Check sheet for the modelled part. Datum: model origin and axes. Units: mm. Face numbers are marked on the shaded views. Coordinates: 2 decimals unless noted, no trailing zeros. Write each loop counter-clockwise with the first axis right and the second up, starting at its lowest first coordinate (ties: lowest second). Pieces come first, ordered by that corner, then holes. Notation, with made-up numbers: (-8, 70.5) -> (1, 70.5) arc R24 ccw to (1, 82.5) -> close; hole circle Ø8 at (21.25, 30). An arc over 180 degrees is marked (long way). Put each result on its own line as item: value.
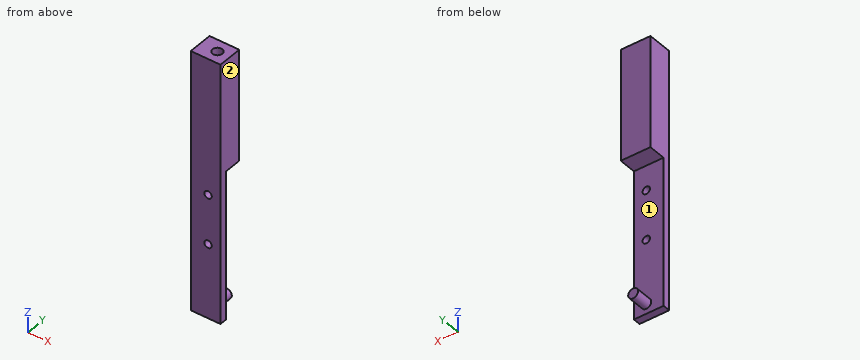
```python
from build123d import *

# Parameters (mm, degrees)
SKETCH1_W               = 10
SKETCH1_H               = 105
BOSS_EXTRUDE1_DEPTH     = 10
SKETCH2_W               = 60
SKETCH2_H               = 13.095712102
CUT_EXTRUDE1_DEPTH      = 10
CUT_EXTRUDE1_DEPTH_BACK = 10
SKETCH3_R               = 2
BOSS_EXTRUDE2_DEPTH     = 7
SKETCH4_R               = 1.5
CUT_EXTRUDE2_DEPTH      = 14
SKETCH5_R               = 2
CUT_EXTRUDE3_DEPTH      = 10
BOSS_EXTRUDE3_DEPTH     = 2


with BuildPart() as part:
    # Sketch1 → Boss-Extrude1 (new body)
    with BuildSketch(Plane(origin=(0, 0, 0), x_dir=(1, 0, 0), z_dir=(0, 1, 0))):
        Rectangle(SKETCH1_W, SKETCH1_H)
    extrude(amount=BOSS_EXTRUDE1_DEPTH)

    # Sketch2 → Cut-Extrude1 (cut, two sides)
    with BuildSketch(Plane(origin=(0, 0, 0), x_dir=(0, 0, -1), z_dir=(1, 0, 0))) as cut_extrude1_sk:
        with Locations((22.5, 9.547856051)):
            Rectangle(SKETCH2_W, SKETCH2_H)
    extrude(amount=CUT_EXTRUDE1_DEPTH, mode=Mode.SUBTRACT)
    extrude(cut_extrude1_sk.sketch, amount=-CUT_EXTRUDE1_DEPTH_BACK, mode=Mode.SUBTRACT)

    # Sketch3 → Boss-Extrude2 (add)
    with BuildSketch(Plane(origin=(0, 3, 0), x_dir=(1, 0, 0), z_dir=(0, 1, 0))):
        with Locations((0, 48.5)):
            Circle(SKETCH3_R)
    extrude(amount=BOSS_EXTRUDE2_DEPTH)

    # Sketch4 → Cut-Extrude2 (cut)
    with BuildSketch(Plane(origin=(0, 0, 0), x_dir=(1, 0, 0), z_dir=(0, 1, 0))):
        with Locations((0, 2.5)):
            Circle(SKETCH4_R)
        with Locations((0, 22.5)):
            Circle(SKETCH4_R)
    extrude(amount=CUT_EXTRUDE2_DEPTH, mode=Mode.SUBTRACT)

    # Sketch5 → Cut-Extrude3 (cut)
    with BuildSketch(Plane.XY.offset(52.5)):
        with Locations((0, 5)):
            Circle(SKETCH5_R)
    extrude(amount=-CUT_EXTRUDE3_DEPTH, mode=Mode.SUBTRACT)

    # Sketch6 → Boss-Extrude3 (add)
    with BuildSketch(Plane.ZY.offset(5)):
        Polygon((7.5, 10), (52.5, 10), (52.5, 0), (-52.5, 0), (-52.5, 3), (7.5, 3), align=None)
    extrude(amount=BOSS_EXTRUDE3_DEPTH)


solid = part.part
```
Q1. Cross-section at A-A (x = 0). Record the cut outline in (y, z).
Recorded:
outline: (0, -52.5) -> (3, -52.5) -> (3, -50.5) -> (10, -50.5) -> (10, -46.5) -> (3, -46.5) -> (3, -24) -> (0, -24) -> close; (0, -21) -> (3, -21) -> (3, -4) -> (0, -4) -> close; (0, -1) -> (3, -1) -> (3, 7.5) -> (10, 7.5) -> (10, 52.5) -> (7, 52.5) -> (7, 42.5) -> (3, 42.5) -> (3, 52.5) -> (0, 52.5) -> close
Q2. Mould release check, pull along Z, two halves, no side actions. Record for the marked faces 1 and 2: released by +Z, released by -Z, zero draft, split by the parting line, or undercut.
Recorded:
face 1: undercut
face 2: zero draft
Q3. Cross-section at D-D (x = -5.25). Record the cut outline in (y, z).
Recorded:
outline: (0, -52.5) -> (3, -52.5) -> (3, 7.5) -> (10, 7.5) -> (10, 52.5) -> (0, 52.5) -> close
Q4. Cross-section at C-C (z = -48.5). Record the cut outline in (x, y), plus the area to 3 significant figures.
Recorded:
outline: (-7, 0) -> (5, 0) -> (5, 3) -> (2, 3) -> (2, 10) -> (-2, 10) -> (-2, 3) -> (-7, 3) -> close
area: 64.0 mm2
Q5. Material ranges on line 1 along Z through (x, y) = (0, 0.6); line 2 along Y through (x, z) = (0, 49.5); line 3 along X through (y, z) = (2.2, -2.5), recorded low to high.
Recorded:
line 1: z = -52.5 to -24, -21 to -4, -1 to 52.5
line 2: y = 0 to 3, 7 to 10
line 3: x = -7 to -1.5, 1.5 to 5
Q6. Depth check by flat-ended pin: P1, Ø5, axis at x = -2.5, z = -8, coming from the -Y side; P2, Ø6, axis at x = -0.5, z = 1, coming from the +Y side; P3, Ø2, axis at x = -1, y = 7, coming from the -Z side. Enter the tip coordinate at first touch or a pass-through.
Recorded:
P1: stops at y = 0
P2: stops at y = 3
P3: stops at z = -50.5
Q7. Cross-section at B-B (z = -22.5). Record the cut outline in (x, y).
Recorded:
outline: (-7, 0) -> (-1.5, 0) -> (-1.5, 3) -> (-7, 3) -> close; (1.5, 0) -> (5, 0) -> (5, 3) -> (1.5, 3) -> close
